Read the model definition and answer for the solid it produces. Units are mm, in the model's axes. A direction names the side the tool comes from. Round coordinates to 2 decimals unless told otherwise and drop trailing zeros. Loops run counter-clockwise (first coordinate to the right, second up) from the corner with the lowest first, then second, coordinate; pieces in that order, holes last. Notation, with made-up numbers: M 89,74.25 L 132,74.25 A25 cw 132,90.25 Z; hole C 72.25,27.25 d10. An arc over 180 degrees is marked long. Answer as CSV lines item,"result".
```python
from build123d import *

# Parameters (mm, degrees)
F0_W     = 203.2
F0_H     = 127
F1_DEPTH = 127
F3_DEPTH = 101.6
F4_SIZE2 = 101.6
F4_SIZE  = 76.2
F5_R     = 5.08
F6_R     = 15.24
F7_DEPTH = 1270
F8_R     = 15.24
F9_DEPTH = 12903.2


with BuildPart() as f1:
    # F0 (on Front) → F1 (new body)
    with BuildSketch(Plane.XZ):
        with Locations((20.8130544846, 1.564221409)):
            Rectangle(F0_W, F0_H)
    extrude(amount=F1_DEPTH)

    # F2 (on face) → F3 (cut)
    with BuildSketch(Plane.XZ.offset(127)):
        Polygon((122.4130544846, 65.064221409), (20.8130544846, 65.064221409), (20.8130544846, 0), (-17.2869455154, 0), (-17.2869455154, -61.935778591), (122.4130544846, -61.935778591), align=None)
    extrude(amount=-F3_DEPTH, mode=Mode.SUBTRACT)

    # F4
    f4_edges = [f1.edges().sort_by_distance(p)[0] for p in [
        (122.413054, -12.7, 65.064221),
    ]]
    f4_side = f1.faces().sort_by_distance((-13.053612, -55.033333, 65.064221))[0]
    chamfer(f4_edges, length=F4_SIZE, length2=F4_SIZE2, reference=f4_side)

    # F5
    f5_edges = [f1.edges().sort_by_distance(p)[0] for p in [
        (-29.986946, -127, 65.064221),
        (20.813054, -76.2, 65.064221),
        (20.813054, -25.4, 32.532111),
        (20.813054, -76.2, 0),
        (1.763054, -127, 0),
        (20.813054, -127, 32.532111),
        (-17.286946, -127, -30.967889),
        (-49.036946, -127, -61.935779),
        (-17.286946, -76.2, -61.935779),
        (-17.286946, -25.4, -30.967889),
        (-17.286946, 0, 65.064221),
        (-80.786946, -63.5, 65.064221),
        (-80.786946, -127, 1.564221),
        (-80.786946, -63.5, -61.935779),
        (20.813054, 0, -61.935779),
        (-80.786946, 0, 1.564221),
        (52.563054, -25.4, -61.935779),
        (33.513054, -25.4, 65.064221),
        (1.763054, -25.4, 0),
    ]]
    fillet(f5_edges, radius=F5_R)

    # F6 (on face) → F7 (cut)
    with BuildSketch(Plane.XZ.offset(25.4)):
        with Locations((38.5930544846, -16.215778591)):
            Circle(F6_R)
    extrude(amount=-F7_DEPTH, mode=Mode.SUBTRACT)

    # F8 (on face) → F9 (cut)
    with BuildSketch(Plane.XY.offset(65.064221409)):
        with Locations((-39.8652739823, -58.7147325277)):
            Circle(F8_R)
    extrude(amount=-F9_DEPTH, mode=Mode.SUBTRACT)


solid = f1.part
```
1) Find section C-C, the plane y = -33. Give the vertices of the cut face in (x, z).
Evaluation:
outline,"M -80.79,-56.86 A5.08 ccw -75.71,-61.94 L -22.37,-61.94 A5.08 ccw -17.29,-56.86 L -17.29,0 L 15.73,0 A5.08 ccw 20.81,5.08 L 20.81,59.98 A5.08 ccw 15.73,65.06 L -75.71,65.06 A5.08 ccw -80.79,59.98 Z"
2) Find section D-D, the plane z = 11.5. Give the vertices of the cut face in (x, y), then the cut area to 3 significant figures.
Evaluation:
outline,"M -80.79,-121.92 A5.08 ccw -75.71,-127 L 15.73,-127 A5.08 ccw 20.81,-121.92 L 20.81,-30.48 A5.08 cw 25.89,-25.4 L 86.39,-25.4 L 86.39,0 L -75.71,0 A5.08 ccw -80.79,-5.08 Z; hole C -39.87,-58.71 d30.48"
area,"13,800 mm^2"
3) Each of these flat-tipped pins is pushed along its axis until it touches: P1, Ø1, axis at y = -14.5, z = -35.5, coming from the +X side; P2, Ø16.5, axis at x = -6.5, y = -74.5, coming from the -Z side; P3, Ø3, axis at x = 56.5, z = 34.5, coming from the -Y side; P4, Ø2, axis at x = 77, z = -18.5, coming from the +Y side. Where does it stop, or does it pass through?
Evaluation:
P1,"stops at x = 122.01"
P2,"stops at z = 0"
P3,"stops at y = -25.4"
P4,"stops at y = 0"
4) Find section A-A, the plane z = -25.5. Give the vertices of the cut face in (x, y), then the cut area to 3 significant figures.
Evaluation:
outline,"M -80.79,-121.92 A5.08 ccw -75.71,-127 L -22.37,-127 A5.08 ccw -17.29,-121.92 L -17.29,-30.48 A5.08 cw -12.21,-25.4 L 26.51,-25.4 L 26.51,0 L -75.71,0 A5.08 ccw -80.79,-5.08 Z; M 50.68,-25.4 L 114.14,-25.4 L 114.14,0 L 50.68,0 Z; hole C -39.87,-58.71 d30.48"
area,"10,000 mm^2"
5) A tool of negligible diameter and unlimited length cuts with its end or side. For faces 5 (the cylindrical face through (37.79, -23.87, 63.62)), 6 (the cylindrical face through (24.74, -1.45, -60.41)), 7 (the cylindrical face through (-3.584, -125.551, 1.528)), from which of +Z, -Z, +X, -X, +Y, -Y can it reach the whole face along a straight path? Write none if from no direction.
Evaluation:
face 5,"+Z, +X, -Y"
face 6,"-Z, +X, -X, +Y"
face 7,"-Z, +X, -Y"
6) Straight lines are drawn through the part: line 1 (Y direction, x = 7.5, z = -25); line 2 (Z direction, x = -1, y = -93); line 3 (Z direction, x = 27.5, y = -22.5). For each, find the intervals that lie inside material, in ascending order.
Evaluation:
line 1,"y = -25.4 to 0"
line 2,"z = 0 to 65.06"
line 3,"z = -61.44 to -26.67, -5.77 to 64.57"
7) Find section B-B, the plane x = 32. Give the vertices of the cut face in (y, z), then the cut area to 3 significant figures.
Evaluation:
outline,"M -25.4,-56.86 A5.08 ccw -20.32,-61.94 L -5.08,-61.94 A5.08 ccw 0,-56.86 L 0,-29.96 L -25.4,-29.96 Z; M -25.4,-2.48 L 0,-2.48 L 0,59.98 A5.08 ccw -5.08,65.06 L -20.32,65.06 A5.08 ccw -25.4,59.98 Z"
area,"2,510 mm^2"
8) Determine the mould class of faces 1 (the cylindrical face through (-79.26, -1.45, 2.38)), 2 (the cylindrical face through (-51.96, -67.99, 2.45)), 3 (the cylindrical face through (-1.008, -26.849, -1.528)), 4 (the cylindrical face through (22.34, -26.85, 32.15)) for opening direction X: released by +X, released by -X, zero draft, split by the parting line, or undercut.
Evaluation:
face 1,"released by -X"
face 2,"undercut"
face 3,"zero draft"
face 4,"released by +X"
